Source: CAD feature listing. Evaluate the final solid. Frame: model axes, mm. Give positions to 0.01 mm unless a question says otherwise; leave off trailing zeros. Write each loop counter-clockwise with the first axis right and the second up, starting at its lowest first coordinate (ties: lowest second). Pieces come first, ordered by that corner, then holes. Notation, with made-up numbers: (-32, 45.5) - (-3, 45.5) arc R30 cw to (-3, 75.5) - close; hole circle Ø7 at (-36.5, 62.5). An arc over 180 degrees is marked (long way). One line per question, with ' | ' between items. Start each with the question number.
(1) Section C-C, the plane y = 3.5. State how many separate pieces and enclosed holes the cut face has, plus the area to 3 significant figures.
(2) Section B-B, the plane z = -190.5. Return loops of the section in (x, y) (3 decimals).
(3) Section A-A, the plane x = -26.5. Return loops of the section in (y, z) (3 decimals).
(4) Ray query, line 1 (X direction, y = 1.5, z = -158.75) (3 decimals); line 2 (Z direction, x = -30, y = 1) (3 decimals); line 3 (Z direction, x = -87, y = 4.75) (3 decimals). Return the intervals inside material, ascending. Write a range as [from, to].
(5) Pin query (flat end, axial travel): pin 1 (6 mm diameter, centred on x = 12.7, z = -6.35, fed in from -Y); pin 2 (4 mm diameter, centred on x = 12.7, z = -171.45, fed in from -Y); pin 3 (3 mm diameter, centred on y = 2.5, z = -114.5, fed in from +X) (3 decimals). Return the tip coordinate at first contact, or that it passes through.
(6) Section D-D, the plane z = -158.75. Return loops of the section in (x, y) (3 decimals).
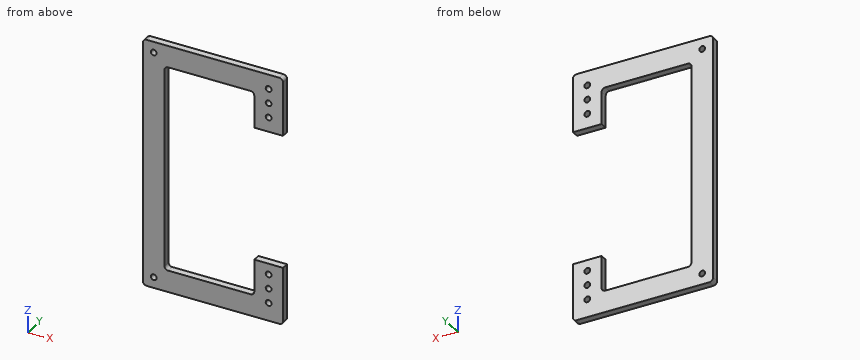
Autodesk Inventor part; units mm, degrees
ref_plane "YZ Plane" through (0, 0, 0) normal (1, 0, 0) x (0, 1, 0)
ref_plane "XZ Plane" through (0, 0, 0) normal (0, 1, 0) x (-1, 0, 0)
ref_plane "XY Plane" through (0, 0, 0) normal (0, 0, 1) x (1, 0, 0)
sketch "Sketch1" plane through (0, 0, 0) normal (0, 1, 0) x (-1, 0, 0)
  line L0 (0, 0) -> (79.375, 0)
  line L1 (79.375, 0) -> (79.375, 19.05) construction
  line L2 (79.375, 19.05) -> (0, 19.05)
  line L3 (0, 19.05) -> (0, 0) construction
  line L4 (79.375, 19.05) -> (98.425, 19.05)
  line L5 (98.425, 19.05) -> (98.425, -200.025)
  line L6 (98.425, -200.025) -> (79.375, -200.025)
  line L7 (79.375, -200.025) -> (79.375, 19.05)
  line L8 (79.375, -200.025) -> (0, -200.025)
  line L9 (0, -200.025) -> (0, -180.975) construction
  line L10 (0, -180.975) -> (79.375, -180.975)
  line L11 (79.375, -180.975) -> (79.375, -200.025) construction
  line L12 (0, 0) -> (-25.4, 0) construction
  line L13 (-25.4, 0) -> (-25.4, 19.05)
  line L14 (-25.4, 19.05) -> (0, 19.05)
  line L15 (0, 19.05) -> (0, 0)
  line L16 (0, -180.975) -> (-25.4, -180.975) construction
  line L17 (-25.4, -180.975) -> (-25.4, -200.025)
  line L18 (-25.4, -200.025) -> (0, -200.025)
  line L19 (0, -200.025) -> (0, -180.975) construction
  circle A0 centre (-12.7, 6.35) radius 2.54 construction
  circle A1 centre (-12.7, -187.325) radius 2.54 construction
  circle A2 centre (88.9, -190.5) radius 2.54 construction
  circle A3 centre (88.9, 9.525) radius 2.54 construction
  line L20 (0, -180.975) -> (-25.4, -180.975) construction
  line L21 (-25.4, -180.975) -> (-25.4, -149.225)
  line L22 (-25.4, -149.225) -> (0, -149.225)
  line L23 (0, -149.225) -> (0, -180.975)
  line L24 (0, -180.975) -> (-25.4, -149.225) construction
  line L25 (-25.4, -180.975) -> (0, -149.225) construction
  line L26 (0, -31.75) -> (-25.4, -31.75)
  line L27 (-25.4, -31.75) -> (-25.4, 0)
  line L28 (-25.4, 0) -> (0, 0) construction
  line L29 (0, 0) -> (0, -31.75)
  line L30 (0, -31.75) -> (-25.4, 0) construction
  line L31 (-25.4, -31.75) -> (0, 0) construction
  point P0 (79.375, 0)
  point P1 (79.375, -180.975)
  point P2 (0, -200.025)
  point P3 (79.375, -190.5)
  point P4 (0, -200.025)
  point P5 (-12.7, -165.1)
  point P6 (-12.7, -15.875)
  dimension "d0" = 79.375
  dimension "d1" = 19.05
  dimension "d3" = 19.05
  dimension "d4" = 79.375
  dimension "d5" = 19.05
  dimension "d8" = 180.975
  dimension "d9" = 25.4
  dimension "d10" = 19.05
  dimension "d11" = 25.4
  dimension "d12" = 19.05
  dimension "d17" = 5.08
  dimension "d18" = 6.35
  dimension "d20" = 5.08
  dimension "d21" = 12.7
  dimension "d23" = 12.7
  dimension "d38" = 5.08
  dimension "d39" = 9.525
  dimension "d40" = 9.525
  dimension "d41" = 5.08
  dimension "d42" = 9.525
  dimension "d43" = 9.525
  dimension "d52" = 12.7
  dimension "d53" = 25.4
  dimension "d54" = 50.8
  dimension "d55" = 50.8
  dimension "d56" = 25.4
extrude "Extrusion1" add sketch "Sketch1" along normal blind 6.35
hole "Hole3" at (-88.9, 0, -190.5) at (-88.9, 0, 9.525) direction (0, 1, 0) diameter 5.1054 end through all
fillet "Fillet1" radius 3.175 8 edges at (-98.425, 3.175, -200.025) (25.4, 3.175, -200.025) (-79.375, 3.175, -180.975) (-79.375, 3.175, 0) (-98.425, 3.175, 19.05) (25.4, 3.175, 19.05) (0, 3.175, 0) (0, 3.175, -180.975)
sketch "Sketch3" plane through (0, 6.35, 0) normal (0, 1, 0) x (1, 0, 0)
  line L0 (-95.25, -19.05) -> (22.225, -19.05) construction
  line L1 (25.4, -15.875) -> (25.4, 31.75) construction
  point P0 (0, 0)
  point P1 (12.7, -6.35)
  point P2 (12.7, 6.35)
  point P3 (12.7, 19.05)
  point P4 (12.7, 31.75)
  point P5 (12.7, 44.45)
  point P6 (12.7, 57.15)
  point P7 (12.7, 69.85)
  point P8 (12.7, 82.55)
  point P9 (12.7, 95.25)
  point P10 (12.7, 107.95)
  point P11 (12.7, 120.65)
  point P12 (12.7, 133.35)
  point P13 (12.7, 146.05)
  point P14 (12.7, 158.75)
  point P15 (12.7, 171.45)
  point P16 (12.7, 184.15)
  dimension "d57" = 12.7
  dimension "d58" = 12.7
  dimension "d61" = 12.7
hole "Hole4" at (12.7, 6.35, 6.35) at (12.7, 6.35, -6.35) at (12.7, 6.35, -19.05) at (12.7, 6.35, -44.45) at (12.7, 6.35, -57.15) at (12.7, 6.35, -69.85) at (12.7, 6.35, -82.55) at (12.7, 6.35, -95.25) at (12.7, 6.35, -107.95) at (12.7, 6.35, -120.65) at (12.7, 6.35, -133.35) at (12.7, 6.35, -146.05) at (12.7, 6.35, -158.75) at (12.7, 6.35, -171.45) at (12.7, 6.35, -184.15) direction (0, -1, 0) diameter 5.1054 end through all
equation "\"d4\" = d0"
properties part number "DB1-009" material "Aluminum 6061"
Check sheet entries:
1) separate pieces: 1 | enclosed holes: 8 | area: 9,610 mm²
2) outline: (-98.425, 0) - (-91.453, 0) - (-91.453, 6.35) - (-98.425, 6.35) - close; (-86.347, 0) - (25.4, 0) - (25.4, 6.35) - (-86.347, 6.35) - close
3) outline: (0, -200.025) - (6.35, -200.025) - (6.35, -180.975) - (0, -180.975) - close; (0, 0) - (6.35, 0) - (6.35, 19.05) - (0, 19.05) - close
4) line 1: [-98.425, -79.375], [0, 10.147], [15.253, 25.4] | line 2: [-200.025, -180.975], [0, 19.05] | line 3: [-200.025, -192.205], [-188.795, 7.82], [11.23, 19.05]
5) pin 1: y = 0 | pin 2: through | pin 3: x = -79.375
6) outline: (-98.425, 0) - (-79.375, 0) - (-79.375, 6.35) - (-98.425, 6.35) - close; (0, 0) - (10.147, 0) - (10.147, 6.35) - (0, 6.35) - close; (15.253, 0) - (25.4, 0) - (25.4, 6.35) - (15.253, 6.35) - close
